Geometry: final body of the model. Coordinates: model frame, mm. A direction names the side the tool comes from. Coordinates: 2 decimals unless noted, no trailing zeros. Write each loop counter-clockwise with the first axis right and the second up, starting at its lowest first coordinate (ties: lowest second). Pieces come first, ordered by that corner, then holes. Notation, with made-up numbers: (-1, 2) -> (29, 2) arc R23 cw to (29, 17) -> close; hole circle Ø1 at (-37, -17.5). An arc over 180 degrees is marked (long way). One line per item, written item: value.
Autodesk Inventor part; units mm, degrees
ref_plane "YZ Plane" through (0, 0, 0) normal (1, 0, 0) x (0, 1, 0)
ref_plane "XZ Plane" through (0, 0, 0) normal (0, 1, 0) x (-1, 0, 0)
ref_plane "XY Plane" through (0, 0, 0) normal (0, 0, 1) x (1, 0, 0)
sketch "Sketch1" plane through (0, 0, 0) normal (0, 1, 0) x (-1, 0, 0)
  line L0 (0, 0) -> (52.07, 0)
  line L1 (52.07, 0) -> (52.07, 26.67)
  line L2 (52.07, 26.67) -> (0, 26.67)
  line L3 (0, 26.67) -> (0, 0)
  line L4 (-12.7, 39.37) -> (64.77, 39.37)
  line L5 (64.77, 39.37) -> (64.77, -12.7)
  line L6 (64.77, -12.7) -> (-12.7, -12.7)
  line L7 (-12.7, -12.7) -> (-12.7, 39.37)
  dimension "d0" = 26.67
  dimension "d1" = 52.07
  dimension "d2" = 12.7
  dimension "d3" = 12.7
  dimension "d4" = 12.7
  dimension "d5" = 12.7
extrude "Extrusion1" add sketch "Sketch1" along normal blind 127
sketch "Sketch2" plane through (0, 0, 0) normal (0, -1, 0) x (1, 0, 0)
  line L0 (0, 0) -> (-52.07, 0)
  line L1 (-52.07, 0) -> (-52.07, 26.67)
  line L2 (-52.07, 26.67) -> (0, 26.67)
  line L3 (0, 26.67) -> (0, 0)
extrude "Extrusion2" add sketch "Sketch2" against normal blind 5.08
properties part number "HammerStick Sleeve"
(1) Reachability of faces 1 (the flat face through (12.7, 63, 13)), 2 (the flat face through (-26, 65, 26.67)) from +Z, -Z, +X, -X, +Y, -Y: full face, straight path, thin tool, end or side. Return the list, or none.
Responses:
face 1: +Z, -Z, +X, +Y, -Y
face 2: +Y
(2) Section B-B (z = 2.5). Return the cut outline in (x, y).
Responses:
outline: (-64.77, 0) -> (12.7, 0) -> (12.7, 127) -> (0, 127) -> (0, 5.08) -> (-52.07, 5.08) -> (-52.07, 127) -> (-64.77, 127) -> close
(3) Section A-A (y = 99.5). Return the cut outline in (x, z), then the cut area to 3 significant figures.
Responses:
outline: (-64.77, -12.7) -> (12.7, -12.7) -> (12.7, 39.37) -> (-64.77, 39.37) -> close; hole (-52.07, 0) -> (0, 0) -> (0, 26.67) -> (-52.07, 26.67) -> close
area: 2,650 mm2
(4) Section C-C (x = -23). Return the cut outline in (y, z), then the cut area to 3 significant figures.
Responses:
outline: (0, -12.7) -> (127, -12.7) -> (127, 0) -> (5.08, 0) -> (5.08, 26.67) -> (127, 26.67) -> (127, 39.37) -> (0, 39.37) -> close
area: 3,360 mm2
(5) Pull-direction query (Z, two-part tool) for faces 3 (the flat face through (-25, 63, 39.37)), 4 (the flat face through (0, 65, 14)), 5 (the flat face through (-64.77, 63, 14)), 6 (the flat face through (-27, 63, -12.7)); classes: released by +Z, released by -Z, zero draft, split by the parting line, or undercut.
Responses:
face 3: released by +Z
face 4: undercut
face 5: zero draft
face 6: released by -Z
(6) Line query: line 1 (X direction, y = 79.5, z = 23); line 2 (Z direction, x = -22, y = 37); line 3 (Y direction, x = -32.5, z = 12). Output: solid intervals per line, ascending. Write a range as [from, to].
Responses:
line 1: x = [-64.77, -52.07], [0, 12.7]
line 2: z = [-12.7, 0], [26.67, 39.37]
line 3: y = [0, 5.08]
